Part model, mm, in its own coordinate system. A direction names the side the tool comes from. Give positions to 0.01 mm unless a question says otherwise; leave off trailing zeros. Order: outer loops, then holes, each group sorted by start corner. A loop starts at its lowest first (then second) coordinate and runs counter-clockwise, first axis right, second up. Notation, with made-up numbers: M 62.5,6.25 L 102.5,6.25 A14 ccw 102.5,25.25 Z; hole C -26.75,51 d10. An arc over 180 degrees is marked long. Return JSON: item names as keys, results as strings.
Autodesk Inventor part; units mm, degrees
ref_plane "YZ Plane" through (0, 0, 0) normal (1, 0, 0) x (0, 1, 0)
ref_plane "XZ Plane" through (0, 0, 0) normal (0, 1, 0) x (-1, 0, 0)
ref_plane "XY Plane" through (0, 0, 0) normal (0, 0, 1) x (1, 0, 0)
sketch "Skizze1" plane through (0, 0, 0) normal (1, 0, 0) x (0, 1, 0)
  line L0 (8, 460) -> (-8, 460)
  line L1 (-10, 458) -> (-10, 347)
  line L2 (-8, 345) -> (8, 345)
  line L3 (10, 347) -> (10, 458)
  line L4 (8, 345) -> (-8, 345)
  line L5 (-10, 343) -> (-10, 232)
  line L6 (-8, 230) -> (8, 230)
  line L7 (10, 232) -> (10, 343)
  line L8 (8, 230) -> (-8, 230)
  line L9 (-10, 228) -> (-10, 117)
  line L10 (-8, 115) -> (8, 115)
  line L11 (10, 117) -> (10, 228)
  line L12 (8, 115) -> (-8, 115)
  line L13 (-10, 113) -> (-10, 2)
  line L14 (-8, 0) -> (8, 0)
  line L15 (10, 2) -> (10, 113)
  line L16 (8, 0) -> (-8, 0)
  line L17 (-10, -2) -> (-10, -113)
  line L18 (-8, -115) -> (8, -115)
  line L19 (10, -113) -> (10, -2)
  line L20 (8, -115) -> (-8, -115)
  line L21 (-10, -117) -> (-10, -228)
  line L22 (-8, -230) -> (8, -230)
  line L23 (10, -228) -> (10, -117)
  line L24 (8, -230) -> (-8, -230)
  line L25 (-10, -232) -> (-10, -343)
  line L26 (-8, -345) -> (8, -345)
  line L27 (10, -343) -> (10, -232)
  line L28 (10, -343) -> (8, -345)
  line L29 (10, -232) -> (8, -230)
  line L30 (10, -228) -> (8, -230)
  line L31 (10, -117) -> (8, -115)
  line L32 (8, -115) -> (10, -113)
  line L33 (10, -2) -> (8, 0)
  line L34 (8, 0) -> (10, 2)
  line L35 (10, 113) -> (8, 115)
  line L36 (8, 115) -> (10, 117)
  line L37 (10, 228) -> (8, 230)
  line L38 (10, 232) -> (8, 230)
  line L39 (10, 343) -> (8, 345)
  line L40 (10, 347) -> (8, 345)
  line L41 (10, 458) -> (8, 460)
  line L42 (-8, -345) -> (-10, -343)
  line L43 (-10, -232) -> (-8, -230)
  line L44 (-10, -228) -> (-8, -230)
  line L45 (-10, -117) -> (-8, -115)
  line L46 (-10, -113) -> (-8, -115)
  line L47 (-10, -2) -> (-8, 0)
  line L48 (-10, 2) -> (-8, 0)
  line L49 (-10, 113) -> (-8, 115)
  line L50 (-10, 117) -> (-8, 115)
  line L51 (-10, 343) -> (-8, 345)
  line L52 (-10, 347) -> (-8, 345)
  line L53 (-8, 460) -> (-10, 458)
  line L54 (8, -345) -> (-8, -345)
  line L55 (-10, -347) -> (-10, -458)
  line L56 (-8, -460) -> (8, -460)
  line L57 (10, -458) -> (10, -347)
  line L58 (8, -345) -> (10, -347)
  line L59 (10, -458) -> (8, -460)
  line L60 (-8, -460) -> (-10, -458)
  line L61 (-10, -347) -> (-8, -345)
  line L62 (-8, 230) -> (-10, 232)
  line L63 (-8, 230) -> (-10, 228)
  point P0 (0, 115)
  point P1 (10, 460)
  point P2 (-10, 345)
  point P3 (-10, 460)
  point P4 (10, 345)
  point P5 (-10, 230)
  point P6 (-10, 345)
  point P7 (10, 230)
  point P8 (-10, 115)
  point P9 (-10, 230)
  point P10 (10, 115)
  point P11 (-10, 0)
  point P12 (-10, 115)
  point P13 (10, 0)
  point P14 (-10, -115)
  point P15 (-10, 0)
  point P16 (10, -115)
  point P17 (-10, -230)
  point P18 (-10, -115)
  point P19 (10, -230)
  point P20 (0, 115)
  point P21 (-10, 230)
  point P22 (-10, 230)
  point P23 (-9, 0)
  point P24 (-9, -115)
  point P25 (-9, -230)
  point P26 (-10, -345)
  point P27 (10, -345)
  point P28 (-10, 0)
  point P29 (-10, 0)
  point P30 (-10, 0)
  point P31 (-10, 115)
  point P32 (-10, 115)
  point P33 (-10, 345)
  point P34 (-10, 345)
  point P35 (-8, -115)
  point P36 (-10, -460)
  point P37 (-10, -345)
  point P38 (10, -460)
  point P39 (0, 0)
  point P40 (0, 0)
  dimension "d0" = 20
  dimension "d1" = 115
  dimension "d30" = 2
  dimension "d31" = 2
  dimension "d32" = 2
  dimension "d33" = 2
  dimension "d34" = 2
  dimension "d35" = 2
  dimension "d36" = 2
  dimension "d37" = 2
  dimension "d38" = 2
  dimension "d39" = 2
  dimension "d40" = 2
  dimension "d41" = 2
  dimension "d42" = 2
  dimension "d43" = 2
  dimension "d44" = 2
  dimension "d45" = 2
  dimension "d46" = 2
  dimension "d47" = 2
  dimension "d48" = 2
  dimension "d49" = 2
  dimension "d50" = 2
  dimension "d51" = 2
  dimension "d52" = 2
  dimension "d53" = 2
  dimension "d54" = 2
  dimension "d55" = 2
  dimension "d56" = 2
  dimension "d57" = 2
  dimension "d58" = 2
  dimension "d59" = 2
  dimension "d60" = 2
  dimension "d61" = 2
  dimension "d62" = 2
  dimension "d63" = 2
  dimension "d64" = 2
  dimension "d65" = 2
  dimension "d66" = 2
  dimension "d67" = 2
  dimension "d68" = 2
  dimension "d69" = 2
  dimension "d70" = 2
  dimension "d71" = 2
  dimension "d72" = 2
  dimension "d73" = 2
  dimension "d74" = 2
  dimension "d75" = 2
  dimension "d76" = 2
  dimension "d77" = 2
  dimension "d78" = 2
  dimension "d79" = 2
  dimension "d80" = 2
  dimension "d81" = 2
  dimension "d90" = 2
  dimension "d91" = 2
  dimension "d92" = 2
  dimension "d93" = 2
  dimension "d94" = 2
  dimension "d95" = 2
  dimension "d96" = 2
  dimension "d97" = 2
  dimension "d102" = 2
  dimension "d103" = 2
extrude "Extrusion1" add sketch "Skizze1" along normal blind 450 and the other way blind 400 contours L41 L3 L40 L2 L52 L1 L53 L0
extrude "Extrusion3" add sketch "Skizze1" along normal blind 475 and the other way blind 425 contours L37 L11 L36 L10 L50 L9 L63 L6
extrude "Extrusion2" add sketch "Skizze1" along normal blind 500 and the other way blind 350 contours L39 L7 L38 L6 L62 L5 L51 L2
extrude "Extrusion4" add sketch "Skizze1" along normal blind 425 and the other way blind 375 contours L35 L15 L34 L14 L48 L13 L49 L10
extrude "Extrusion5" add sketch "Skizze1" along normal blind 460 and the other way blind 400 contours L33 L19 L32 L18 L46 L17 L47 L14
extrude "Extrusion6" add sketch "Skizze1" along normal blind 440 and the other way blind 425 contours L31 L23 L30 L22 L44 L21 L45 L18
extrude "Extrusion7" add sketch "Skizze1" along normal blind 475 and the other way blind 400 contours L29 L27 L28 L26 L42 L25 L43 L22
extrude "Extrusion9" add sketch "Skizze1" along normal blind 450 and the other way blind 450 contours L58 L57 L59 L56 L60 L55 L61 L26
sketch "Skizze2" plane through (-400, 10, 458) normal (0, 1, 0) x (1, 0, 0)
  line L0 (747.5, 33) -> (787.5, 33)
  line L1 (787.5, 33) -> (787.5, 883)
  line L2 (787.5, 883) -> (747.5, 883)
  line L3 (747.5, 883) -> (747.5, 33)
  line L4 (87.5, 33) -> (127.5, 33)
  line L5 (127.5, 33) -> (127.5, 883)
  line L6 (127.5, 883) -> (87.5, 883)
  line L7 (87.5, 883) -> (87.5, 33)
  line L8 (87.5, 33) -> (787.5, 33) construction
  line L9 (787.5, 33) -> (787.5, 883) construction
  line L10 (787.5, 883) -> (87.5, 883) construction
  line L11 (87.5, 883) -> (87.5, 33) construction
  line L12 (-25, -2) -> (900, -2) construction
  line L13 (900, -2) -> (900, 918) construction
  line L14 (900, 918) -> (-25, 918) construction
  line L15 (-25, 918) -> (-25, -2) construction
  line L16 (0, -2) -> (850, -2) construction
  line L17 (-25, 230) -> (-25, 341) construction
  line L18 (900, 226) -> (900, 115) construction
  line L19 (0, 803) -> (875, 803) construction
  line L20 (-25, 458) -> (900, 458) construction
  line L21 (0, 803) -> (875, 803) construction
  line L22 (437.5, -2) -> (437.5, 918) construction
  line L23 (-50, 918) -> (850, 918)
  point P0 (400, 458)
  point P1 (87.5, 458)
  point P2 (437.5, 33)
  dimension "d82" = 40
  dimension "d83" = 40
  dimension "d84" = 850
  dimension "d85" = 700
extrude "Extrusion8" add sketch "Skizze2" along normal blind 60
equation "\"d83\" = d82"
properties part number "Backboard" material "Holz (Birke)"
Q1. Pin check, flat tips, straight feed: pin 1 (6 mm diameter, centred on y = -3.5, z = 58.5, fed in from +X); pin 2 (2 mm diameter, centred on x = -287, z = 230.5, fed in from -Y); pin 3 (22 mm diameter, centred on y = -4.5, z = 167, fed in from +X). Stop position of each tip, or through.
Established:
{"pin 1": "stops at x = 425", "pin 2": "stops at y = -9.5", "pin 3": "stops at x = 475"}
Q2. Probe line 1 along Z through (x, y) = (-387.5, -4.5); line 2 along X through (y, z) = (26, 110); line 3 along Z through (x, y) = (375.5, 48). List the from-to ranges inside material, lowest first.
Established:
{"line 1": "z = -460 to 0, 115 to 230, 345 to 460", "line 2": "x = -312.5 to -272.5, 347.5 to 387.5", "line 3": "z = -425 to 425"}
Q3. Band-saw the part on B-B (z = -251). Give the cut face in (x, y).
Established:
{"outline": "M -400,-10 L 475,-10 L 475,10 L 387.5,10 L 387.5,70 L 347.5,70 L 347.5,10 L -272.5,10 L -272.5,70 L -312.5,70 L -312.5,10 L -400,10 Z"}
Q4. Two-plate mould, pull along Z, no slides. Class faces 1 (the flat face through (-293, 40, 425)), 2 (the flat face through (475, 0, 173)), 3 (the flat face through (425, 0, 58)): +Z half, -Z half, draft (parallel to the pull), parting line (faces both ways), or undercut.
Established:
{"face 1": "+Z half", "face 2": "draft", "face 3": "undercut"}
Q5. 3-axis set-ups, long thin cutter, end or side, ignore diameter. For faces 4 (the flat face through (450, 0, -402)), 5 (the flat face through (-370, 10, 172)), 6 (the flat face through (367, 40, 425)), 7 (the flat face through (33, 10, 287)), 8 (the flat face through (413, 10, -173)): which of +Z, -Z, +X, -X, +Y, -Y reach the whole face in a straight line?
Established:
{"face 4": "-Z, +X, +Y, -Y", "face 5": "+Z, -Z, -X, +Y", "face 6": "+Z, +X, -X, +Y", "face 7": "+Z, -Z, +Y", "face 8": "+Z, -Z, +X, +Y"}
Q6. Band-saw the part on A-A (y = 37.5). Give the cut face in (x, z).
Established:
{"outline": "M -312.5,-425 L -272.5,-425 L -272.5,425 L -312.5,425 Z; M 347.5,-425 L 387.5,-425 L 387.5,425 L 347.5,425 Z"}
Q7. Band-saw the part on C-C (z = 75). Give the cut face in (x, y).
Established:
{"outline": "M -375,-10 L 425,-10 L 425,10 L 387.5,10 L 387.5,70 L 347.5,70 L 347.5,10 L -272.5,10 L -272.5,70 L -312.5,70 L -312.5,10 L -375,10 Z"}
